```python
from build123d import *

# Parameters (mm, degrees)
SKETCH1_W           = 482.6
SKETCH1_H           = 355.6
BOSS_EXTRUDE1_DEPTH = 6.35
SKETCH2_R           = 2.55
CUT_EXTRUDE1_DEPTH  = 600.495156361
FILLET1_R           = 12.7
SKETCH5_R           = 1.5
CUT_EXTRUDE4_DEPTH  = 600.495156361
SKETCH8_W           = 19.05
SKETCH8_H           = 50.8
CUT_EXTRUDE7_DEPTH  = 63.5
CUT_EXTRUDE9_DEPTH  = 6.35
SKETCH12_R          = 14
SKETCH12_W          = 12.7
SKETCH12_H          = 10.884798806
CUT_EXTRUDE11_DEPTH = 63.5
SKETCH13_W          = 220.004592511
SKETCH13_H          = 264.065052174
BOSS_EXTRUDE2_DEPTH = 6.35
SKETCH15_R          = 13.97
CUT_EXTRUDE13_DEPTH = 600.495156361
LPATTERN1_COUNT     = 4
LPATTERN1_PITCH     = 35.56
SKETCH17_W          = 228.6
SKETCH17_H          = 11.43
CUT_EXTRUDE14_DEPTH = 600.495156361
SKETCH18_W          = 19.05
SKETCH18_H          = 50.8
CUT_EXTRUDE15_DEPTH = 600.495156361
SKETCH19_R          = 1.5875
CUT_EXTRUDE16_DEPTH = 600.495156361
SKETCH20_R          = 57.15
CUT_EXTRUDE17_DEPTH = 600.495156361
SKETCH21_R          = 3.175
CUT_EXTRUDE18_DEPTH = 600.495156361


with BuildPart() as part:
    # Sketch1 → Boss-Extrude1 (new body)
    with BuildSketch(Plane(origin=(0, 0, 0), x_dir=(1, 0, 0), z_dir=(0, 1, 0))):
        with Locations((241.3, 177.8)):
            Rectangle(SKETCH1_W, SKETCH1_H)
    extrude(amount=BOSS_EXTRUDE1_DEPTH)

    # Sketch2 → Cut-Extrude1 (cut, through all)
    with BuildSketch(Plane(origin=(0, 6.35, 0), x_dir=(1, 0, 0), z_dir=(0, 1, 0))):
        with Locations(Location((25.4, 330.2, 0), (0, 0, 270))):
            Circle(SKETCH2_R)
        with Locations(Location((241.3, 330.2, 0), (0, 0, 270))):
            Circle(SKETCH2_R)
        with Locations(Location((457.2, 330.2, 0), (0, 0, 270))):
            Circle(SKETCH2_R)
        with Locations(Location((241.3, 25.4, 0), (0, 0, 270))):
            Circle(SKETCH2_R)
        with Locations(Location((457.2, 25.4, 0), (0, 0, 270))):
            Circle(SKETCH2_R)
        with Locations(Location((25.4, 25.4, 0), (0, 0, 270))):
            Circle(SKETCH2_R)
    extrude(amount=-CUT_EXTRUDE1_DEPTH, mode=Mode.SUBTRACT)

    # Fillet1
    fillet1_edges = [part.edges().sort_by_distance(p)[0] for p in [
        (0, 3.175, -355.6),
        (482.6, 3.175, -355.6),
        (482.6, 3.175, 0),
        (0, 3.175, 0),
    ]]
    fillet(fillet1_edges, radius=FILLET1_R)

    # Sketch5 → Cut-Extrude4 (cut, through all)
    with BuildSketch(Plane(origin=(0, 6.35, 0), x_dir=(1, 0, 0), z_dir=(0, 1, 0))):
        with Locations(Location((254, 317.5, 0), (0, 0, 270))):
            Circle(SKETCH5_R)
        with Locations(Location((304.8, 317.5, 0), (0, 0, 270))):
            Circle(SKETCH5_R)
        with Locations(Location((406.4, 317.5, 0), (0, 0, 270))):
            Circle(SKETCH5_R)
        with Locations(Location((457.2, 317.5, 0), (0, 0, 270))):
            Circle(SKETCH5_R)
        with Locations(Location((304.8, 301.498, 0), (0, 0, 270))):
            Circle(SKETCH5_R)
        with Locations(Location((406.4, 301.498, 0), (0, 0, 270))):
            Circle(SKETCH5_R)
        with Locations(Location((457.2, 301.498, 0), (0, 0, 270))):
            Circle(SKETCH5_R)
        with Locations(Location((254, 301.498, 0), (0, 0, 270))):
            Circle(SKETCH5_R)
    cut_extrude4 = extrude(amount=-CUT_EXTRUDE4_DEPTH, mode=Mode.SUBTRACT)

    # Sketch8 → Cut-Extrude7 (cut, symmetric)
    with BuildSketch(Plane(origin=(0, 6.35, 0), x_dir=(1, 0, 0), z_dir=(0, 1, 0))):
        with Locations((200.025, 177.8)):
            Rectangle(SKETCH8_W, SKETCH8_H)
    extrude(amount=CUT_EXTRUDE7_DEPTH, both=True, mode=Mode.SUBTRACT)

    # Sketch10 → Cut-Extrude9 (cut)
    with BuildSketch(Plane(origin=(0, 6.35, 0), x_dir=(1, 0, 0), z_dir=(0, 1, 0))):
        Polygon((109.7915, 301.9425), (20.8788, 301.9425), (20.8788, 297.4467), (25.4, 297.4467), (25.4, 58.1533), (20.8788, 58.1533), (20.8788, 53.6575), (109.7915, 53.6575), (109.7915, 58.1533), (29.8958, 58.1533), (29.8958, 297.4467), (109.7915, 297.4467), align=None)
        Polygon((224.1042, 301.9425), (135.1915, 301.9425), (135.1915, 297.4467), (215.0872, 297.4467), (215.0872, 190.5), (219.583, 190.5), (219.583, 297.4467), (224.1042, 297.4467), align=None)
        Polygon((219.583, 165.1), (215.0872, 165.1), (215.0872, 58.1533), (135.1915, 58.1533), (135.1915, 53.6575), (224.1042, 53.6575), (224.1042, 58.1533), (219.583, 58.1533), align=None)
    extrude(amount=-CUT_EXTRUDE9_DEPTH, mode=Mode.SUBTRACT)

    # Sketch12 → Cut-Extrude11 (cut, symmetric)
    with BuildSketch(Plane(origin=(0, 6.35, 0), x_dir=(1, 0, 0), z_dir=(0, 1, 0))):
        with Locations((50.8, 241.3)):
            Circle(SKETCH12_R)
        with Locations((50.8, 114.3)):
            Circle(SKETCH12_R)
        with Locations((70.04884835, 241.3)):
            Rectangle(SKETCH12_W, SKETCH12_H)
        with Locations((70.04884835, 114.3)):
            Rectangle(SKETCH12_W, SKETCH12_H)
    extrude(amount=CUT_EXTRUDE11_DEPTH, both=True, mode=Mode.SUBTRACT)

    # Sketch13 → Boss-Extrude2 (add)
    with BuildSketch(Plane(origin=(0, 6.35, 0), x_dir=(1, 0, 0), z_dir=(0, 1, 0))):
        with Locations((121.094975677, 181.991146523)):
            Rectangle(SKETCH13_W, SKETCH13_H)
    extrude(amount=-BOSS_EXTRUDE2_DEPTH)

    # Sketch15 → Cut-Extrude13 (cut, through all)
    with BuildSketch(Plane(origin=(0, 6.35, 0), x_dir=(1, 0, 0), z_dir=(0, 1, 0))):
        with Locations(Location((50.8, 241.3, 0), (0, 0, 270))):
            Circle(SKETCH15_R)
        with Locations(Location((50.8, 114.3, 0), (0, 0, 270))):
            Circle(SKETCH15_R)
    extrude(amount=-CUT_EXTRUDE13_DEPTH, mode=Mode.SUBTRACT)

    # LPattern1: Cut-Extrude4 ×4
    with Locations(*[(0, 0, i * LPATTERN1_PITCH) for i in range(1, LPATTERN1_COUNT)]):
        add(cut_extrude4, mode=Mode.SUBTRACT)

    # Sketch17 → Cut-Extrude14 (cut, through all)
    with BuildSketch(Plane(origin=(0, 6.35, 0), x_dir=(1, 0, 0), z_dir=(0, 1, 0))):
        with Locations((355.6, 309.499)):
            Rectangle(SKETCH17_W, SKETCH17_H)
        with Locations((355.6, 273.939)):
            Rectangle(SKETCH17_W, SKETCH17_H)
        with Locations((355.6, 238.379)):
            Rectangle(SKETCH17_W, SKETCH17_H)
        with Locations((355.6, 202.819)):
            Rectangle(SKETCH17_W, SKETCH17_H)
    extrude(amount=-CUT_EXTRUDE14_DEPTH, mode=Mode.SUBTRACT)

    # Sketch18 → Cut-Extrude15 (cut, through all)
    with BuildSketch(Plane(origin=(0, 6.35, 0), x_dir=(1, 0, 0), z_dir=(0, 1, 0))):
        with Locations((200.025, 177.8)):
            Rectangle(SKETCH18_W, SKETCH18_H)
    extrude(amount=-CUT_EXTRUDE15_DEPTH, mode=Mode.SUBTRACT)

    # Sketch19 → Cut-Extrude16 (cut, through all)
    with BuildSketch(Plane(origin=(0, 6.35, 0), x_dir=(1, 0, 0), z_dir=(0, 1, 0))):
        with Locations(Location((182.7, 97.775, 0), (0, 0, 270))):
            Circle(SKETCH19_R)
        with Locations(Location((182.7, 66.025, 0), (0, 0, 270))):
            Circle(SKETCH19_R)
    extrude(amount=-CUT_EXTRUDE16_DEPTH, mode=Mode.SUBTRACT)

    # Sketch20 → Cut-Extrude17 (cut, through all)
    with BuildSketch(Plane(origin=(0, 6.35, 0), x_dir=(1, 0, 0), z_dir=(0, 1, 0))):
        with Locations(Location((116.84, 177.426070104, 0), (0, 0, 270))):
            Circle(SKETCH20_R)
    extrude(amount=-CUT_EXTRUDE17_DEPTH, mode=Mode.SUBTRACT)

    # Sketch21 → Cut-Extrude18 (cut, through all)
    with BuildSketch(Plane(origin=(0, 6.35, 0), x_dir=(1, 0, 0), z_dir=(0, 1, 0))):
        with Locations(Location((116.84, 246.006070104, 0), (0, 0, 270))):
            Circle(SKETCH21_R)
        with Locations(Location((48.26, 177.426070104, 0), (0, 0, 270))):
            Circle(SKETCH21_R)
        with Locations(Location((116.84, 108.846070104, 0), (0, 0, 270))):
            Circle(SKETCH21_R)
        with Locations(Location((165.333383054, 128.93268705, 0), (0, 0, 270))):
            Circle(SKETCH21_R)
        with Locations(Location((165.333383054, 225.919453158, 0), (0, 0, 270))):
            Circle(SKETCH21_R)
    extrude(amount=-CUT_EXTRUDE18_DEPTH, mode=Mode.SUBTRACT)


solid = part.part
```
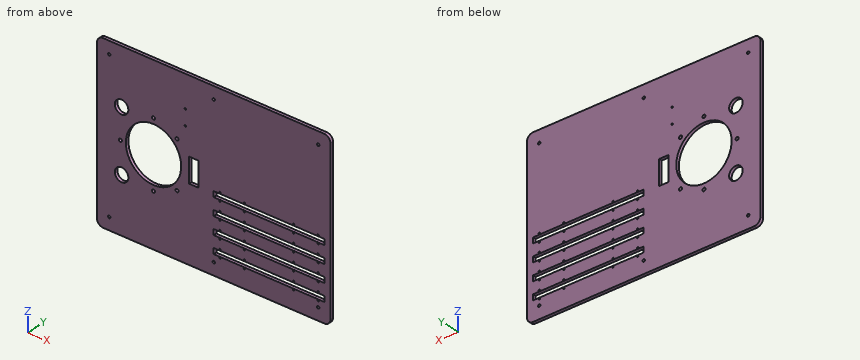
Work out the finished part from the listing and answer in its coordinate system (mm). Give positions to 0.01 mm unless a question says otherwise; leave off trailing zeros. Loops run counter-clockwise (first coordinate to the right, second up) from the corner with the lowest first, then second, coordinate; pieces in that order, holes last. Notation, with made-up numbers: (48, -37) -> (62, -37) arc R20 cw to (62, 2) -> close; hole circle Ø2 at (86.5, -15.75). An arc over 180 degrees is marked (long way). Put each result on its own line as item: value. Start each with the question number.
Item 1: The part is cut by section C-C (z = -163.5). Give the vertices of the cut face in (x, y), then the cut area to 3 significant figures.
Item 2: Find the intervals of material crossed by L1, parallel to Z at x = 368, y = 3.75; L2, parallel to X at y = 2.5, z = -281.94; L3, parallel to Z at x = 50.5, y = 4, in increasing order. Write a range as [from, to].
Item 3: This flat-tipped pin is pushed along its axis until it touches: P1, Ø4.5, axis at x = 241.3, z = -25.4, coming from the +Y side. Where does it stop, or does it pass through?
Item 4: The part is cut by section D-D (y = 1). State how many separate pieces and enclosed holes the cut face has, then the cut area to 3 significant figures.
Item 5: The part is cut by section A-A (x = 441). Give the vertices of the cut face in (y, z), then the cut area to 3 significant figures.
Item 6: The part is cut by section B-B (x = 130.5). Give the vertices of the cut face in (y, z).
Answers below:
1. outline: (0, 0) -> (61.41, 0) -> (61.41, 6.35) -> (0, 6.35) -> close; (172.27, 0) -> (190.5, 0) -> (190.5, 6.35) -> (172.27, 6.35) -> close; (209.55, 0) -> (482.6, 0) -> (482.6, 6.35) -> (209.55, 6.35) -> close
1. area: 2,240 mm2
2. L1: [-355.6, -315.21], [-303.78, -279.65], [-268.22, -244.09], [-232.66, -208.53], [-197.1, 0]
2. L2: [0, 252.5], [255.5, 303.3], [306.3, 404.9], [407.9, 455.7], [458.7, 482.6]
2. L3: [-355.6, -255.27], [-227.33, -179.68], [-175.18, -128.27], [-100.33, 0]
3. P1: through
4. separate pieces: 1
4. enclosed holes: 53
4. area: 148,000 mm2
5. outline: (0, -355.6) -> (6.35, -355.6) -> (6.35, -315.21) -> (0, -315.21) -> close; (0, -303.78) -> (6.35, -303.78) -> (6.35, -279.65) -> (0, -279.65) -> close; (0, -268.22) -> (6.35, -268.22) -> (6.35, -244.09) -> (0, -244.09) -> close; (0, -232.66) -> (6.35, -232.66) -> (6.35, -208.53) -> (0, -208.53) -> close; (0, -197.1) -> (6.35, -197.1) -> (6.35, 0) -> (0, 0) -> close
5. area: 1,970 mm2
6. outline: (0, -355.6) -> (6.35, -355.6) -> (6.35, -232.92) -> (0, -232.92) -> close; (0, -121.93) -> (6.35, -121.93) -> (6.35, 0) -> (0, 0) -> close
